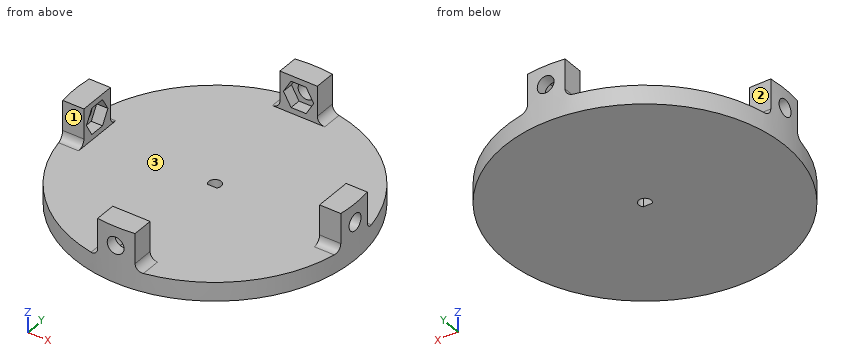
```python
from build123d import *

# Parameters (mm, degrees)
SKETCH_R        = 37.5
PAD_DEPTH       = 5
SKETCH001_W     = 10
SKETCH001_H     = 6
SKETCH001_W_2   = 6
SKETCH001_H_2   = 10
PAD001_DEPTH    = 10
POCKET_DEPTH    = 3
POCKET001_DEPTH = 3
POCKET002_DEPTH = 3
POCKET003_DEPTH = 3
SKETCH006_R     = 2.25
POCKET004_DEPTH = 75
SKETCH007_R     = 2.25
POCKET005_DEPTH = 75
SKETCH008_R     = 1.65
POCKET006_DEPTH = 5
SKETCH009_W     = 2.756733
SKETCH009_H     = 1.311991
PAD002_DEPTH    = 5
SKETCH010_R     = 40
SKETCH010_R_2   = 37.5
POCKET007_DEPTH = 15
FILLET_R        = 2


with BuildPart() as part:
    # Sketch → Pad (new body)
    with BuildSketch(Plane.XY):
        Circle(SKETCH_R)
    extrude(amount=PAD_DEPTH)

    # Sketch001 (on Face3 of Pad) → Pad001 (join)
    with BuildSketch(Plane.XY.offset(5)):
        with Locations((0, 34.5)):
            Rectangle(SKETCH001_W, SKETCH001_H)
        with Locations((0, -34.5)):
            Rectangle(SKETCH001_W, SKETCH001_H)
        with Locations((-34.5, 0)):
            Rectangle(SKETCH001_W_2, SKETCH001_H_2)
        with Locations((34.5, 0)):
            Rectangle(SKETCH001_W_2, SKETCH001_H_2)
    extrude(amount=PAD001_DEPTH)

    # Sketch002 (on Face20 of Pad001) → Pocket (cut)
    with BuildSketch(Plane.YZ.offset(-31.5)):
        Polygon((4.041452, 10), (2.020726, 13.5), (-2.020726, 13.5), (-4.041452, 10), (-2.020726, 6.5), (2.020726, 6.5), align=None)
    extrude(amount=-POCKET_DEPTH, mode=Mode.SUBTRACT)

    # Sketch003 (on Face23 of Pocket) → Pocket001 (cut)
    with BuildSketch(Plane.XZ.offset(-31.5)):
        Polygon((4.041452, 10), (2.020726, 13.5), (-2.020726, 13.5), (-4.041452, 10), (-2.020726, 6.5), (2.020726, 6.5), align=None)
    extrude(amount=-POCKET001_DEPTH, mode=Mode.SUBTRACT)

    # Sketch004 (on Face15 of Pocket001) → Pocket002 (cut)
    with BuildSketch(Plane(origin=(31.5, 0, 0), x_dir=(0, -1, 0), z_dir=(-1, 0, 0))):
        Polygon((4.041452, 10), (2.020726, 13.5), (-2.020726, 13.5), (-4.041452, 10), (-2.020726, 6.5), (2.020726, 6.5), align=None)
    extrude(amount=-POCKET002_DEPTH, mode=Mode.SUBTRACT)

    # Sketch005 (on Face17 of Pocket002) → Pocket003 (cut)
    with BuildSketch(Plane(origin=(0, -31.5, 0), x_dir=(-1, 0, 0), z_dir=(0, 1, 0))):
        Polygon((4.041452, 10), (2.020726, 13.5), (-2.020726, 13.5), (-4.041452, 10), (-2.020726, 6.5), (2.020726, 6.5), align=None)
    extrude(amount=-POCKET003_DEPTH, mode=Mode.SUBTRACT)

    # Sketch006 (on Face12 of Pocket003) → Pocket004 (cut)
    with BuildSketch(Plane.YZ.offset(37.5)):
        with Locations((0, 10)):
            Circle(SKETCH006_R)
    extrude(amount=-POCKET004_DEPTH, mode=Mode.SUBTRACT)

    # Sketch007 (on Face25 of Pocket004) → Pocket005 (cut)
    with BuildSketch(Plane.XZ.offset(37.5)):
        with Locations((0, 10)):
            Circle(SKETCH007_R)
    extrude(amount=-POCKET005_DEPTH, mode=Mode.SUBTRACT)

    # Sketch008 (on Face2 of Pocket005) → Pocket006 (cut)
    with BuildSketch(Plane(origin=(0, 0, 0), x_dir=(1, 0, 0), z_dir=(0, 0, -1))):
        Circle(SKETCH008_R)
    extrude(amount=-POCKET006_DEPTH, mode=Mode.SUBTRACT)

    # Sketch009 (on Face2 of Pocket006) → Pad002 (join)
    with BuildSketch(Plane(origin=(0, 0, 0), x_dir=(1, 0, 0), z_dir=(0, 0, -1))):
        with Locations((-0.025144, 1.755996)):
            Rectangle(SKETCH009_W, SKETCH009_H)
    extrude(amount=-PAD002_DEPTH)

    # Sketch010 (on Face62 of Pad002) → Pocket007 (cut)
    with BuildSketch(Plane(origin=(0, 0, 0), x_dir=(1, 0, 0), z_dir=(0, 0, -1))):
        Circle(SKETCH010_R)
        Circle(SKETCH010_R_2, mode=Mode.SUBTRACT)
    extrude(amount=-POCKET007_DEPTH, mode=Mode.SUBTRACT)

    # Fillet
    fillet_edges = [part.edges().sort_by_distance(p)[0] for p in [
        (5, -34.332586, 5),
        (-5, -34.332586, 5),
        (-34.332586, -5, 5),
        (34.332586, -5, 5),
        (5, 34.332586, 5),
        (34.332586, 5, 5),
        (-34.332586, 5, 5),
        (-5, 34.332586, 5),
    ]]
    fillet(fillet_edges, radius=FILLET_R)


solid = part.part
```
Work out the finished part from the listing and answer in its coordinate system (mm). Face numbers are marked on the shaded views. A direction names the side the tool comes from. Round coordinates to 2 decimals unless told otherwise and drop trailing zeros. Order: outer loops, then holes, each group sorted by start corner. A loop starts at its lowest first (then second) coordinate and runs counter-clockwise, first axis right, second up.
Q1. A cutting plane is placed at D-D, the plane y = 11.5. Determine the outline of the cut face in (x, z).
Solution:
outline: (-35.69, 0) - (35.69, 0) - (35.69, 5) - (-35.69, 5) - close
Q2. A tool of negligible diameter and unlimited length cuts with its end or side. For the marked faces 1, 2 and 3, from which of +Z, -Z, +X, -X, +Y, -Y can it reach the whole face along a straight path? Write none if from no direction.
Solution:
face 1: +Z, +X, -X, -Y
face 2: +Z, +X, -X, +Y
face 3: +Z
Q3. A cutting plane is placed at C-C, the plane z = 11. Count the separate pieces of the cut face and the enclosed holes in it, then the cut area to 3 significant figures.
Solution:
separate pieces: 8
enclosed holes: 0
area: 104 mm2
Q4. A cutting plane is placed at A-A, the plane x = 0. Determine the outline of the cut face in (y, z).
Solution:
outline: (-37.5, 0) - (-1.1, 0) - (-1.1, 5) - (-31.5, 5) - (-31.5, 6.5) - (-34.5, 6.5) - (-34.5, 7.75) - (-37.5, 7.75) - close; (-37.5, 12.25) - (-34.5, 12.25) - (-34.5, 13.5) - (-31.5, 13.5) - (-31.5, 15) - (-37.5, 15) - close; (1.65, 0) - (37.5, 0) - (37.5, 7.75) - (34.5, 7.75) - (34.5, 6.5) - (31.5, 6.5) - (31.5, 5) - (1.65, 5) - close; (31.5, 13.5) - (34.5, 13.5) - (34.5, 12.25) - (37.5, 12.25) - (37.5, 15) - (31.5, 15) - close
Q5. Find the intervals of material crossed by line 1 along Z through (x, y) = (33, -0.5); line 2 along Y through (x, z) = (-33, 10); line 3 along X through (y, z) = (36.9, 10), in increasing order.
Solution:
line 1: z = 0 to 6.5, 13.5 to 15
line 2: y = -5 to -4.04, 4.04 to 5
line 3: x = -5 to -2.25, 2.25 to 5
Q6. Given pin 1 Ø8 at (y, z) = (8.5, 4.5) entering from +X; pin 2 Ø1.5 at (x, y) = (-24, -2) entering from +Z; pin 3 Ø3.5 at (x, y) = (32.5, -1) entering from -Z; pin 4 Ø2.5 at (y, z) = (0, 10) entering from -X, each flat-ended and moving along its own axis, determine where each tip first touches the part or whether it passes through.
Solution:
pin 1: stops at x = 37.23
pin 2: stops at z = 5
pin 3: stops at z = 0
pin 4: passes through
Q7. A cutting plane is placed at B-B, the plane y = 0. Determine the outline of the cut face in (x, z).
Solution:
outline: (-37.5, 0) - (-1.65, 0) - (-1.65, 5) - (-31.5, 5) - (-31.5, 6.5) - (-34.5, 6.5) - (-34.5, 7.75) - (-37.5, 7.75) - close; (-37.5, 12.25) - (-34.5, 12.25) - (-34.5, 13.5) - (-31.5, 13.5) - (-31.5, 15) - (-37.5, 15) - close; (1.65, 0) - (37.5, 0) - (37.5, 7.75) - (34.5, 7.75) - (34.5, 6.5) - (31.5, 6.5) - (31.5, 5) - (1.65, 5) - close; (31.5, 13.5) - (34.5, 13.5) - (34.5, 12.25) - (37.5, 12.25) - (37.5, 15) - (31.5, 15) - close
